Job drawing, mm, ordinate dimensions from the low corner. One solid piece. A direction names the side the tool comes from. Give positions to 0.01 mm unless a question says otherwise; leave off trailing zeros. Order: outer loops, then holes, each group sorted by start corner. A loop starts at its lowest first (then second) coordinate and runs counter-clockwise, first axis right, second up.
Item 1: Band-saw the part on B-B on x = 15. Give the cut face in (y, z) (1 decimal), plus the area to 3 significant figures.
Item 2: Which spindle directions (+Z, -Z, +X, -X, +Y, -Y) get a long thin tool onto all of the face, cutting with end or side? Do the marked faces 1 and 2. Say none if no direction does.
Item 3: Band-saw the part on A-A on x = 10.5. Give the cut face in (y, z) (1 decimal).
Item 4: Flat gauge pins, fed straight in: P1, Ø2, axis at y = 24, z = 16.5, coming from the -X side; P2, Ø10, axis at x = 19.5, y = 10.5, coming from the +Z side; P3, Ø1, axis at x = 7, z = 26.5, coming from the -Y side; P4, Ø1.5, axis at x = 18, y = 19.5, coming from the +Z side. Where does each tip first touch, or does it go through?
Item 5: Wall check: L1, parallel to Y at x = 4, z = 2; L2, parallel to Z at x = 27, y = 19; L3, parallel to Y at x = 35, z = 12. Give the ranges that are in metal, low to high.
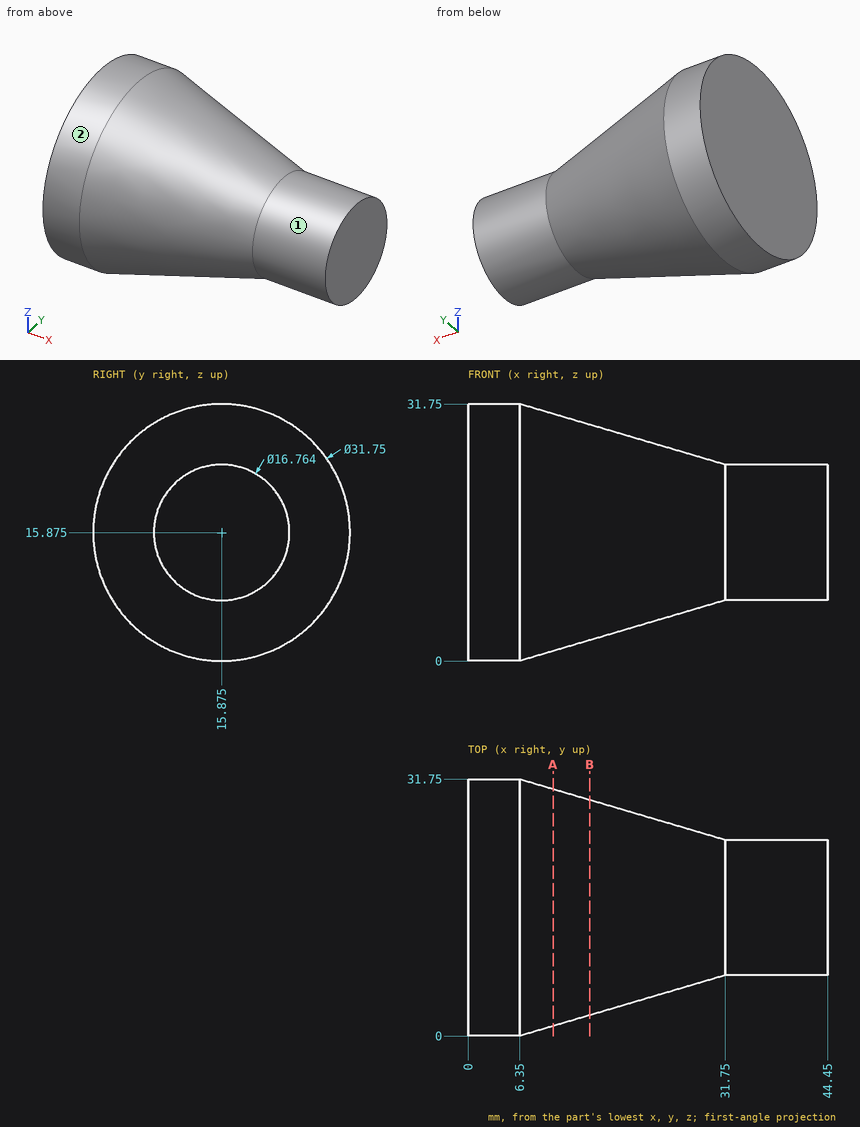
The answers:
1. outline: circle Ø26.6 at (15.9, 15.9)
1. area: 558 mm2
2. face 1: +X
2. face 2: +X, -X
3. outline: circle Ø29.3 at (15.9, 15.9)
4. P1: stops at x = 0
4. P2: stops at z = 28.84
4. P3: stops at y = 3.86
4. P4: stops at z = 28.08
5. L1: y = 8.16 to 23.59
5. L2: z = 6.6 to 25.15
5. L3: y = 8.44 to 23.31
